Autodesk Inventor part; units mm, degrees
ref_plane "YZ Plane" through (0, 0, 0) normal (1, 0, 0) x (0, 1, 0)
ref_plane "XZ Plane" through (0, 0, 0) normal (0, 1, 0) x (-1, 0, 0)
ref_plane "XY Plane" through (0, 0, 0) normal (0, 0, 1) x (1, 0, 0)
sketch "Sketch1" plane through (0, 0, 0) normal (0, 0, 1) x (1, 0, 0)
  circle A0 centre (0, 0) radius 12.2936
  dimension "d0" = 24.5872
extrude "Extrusion1" add sketch "Sketch1" along normal blind 18.796
sketch "Sketch2" plane through (0, 0, 18.796) normal (0, 0, 1) x (1, 0, 0)
  circle A0 centre (0, 0) radius 12.2936
  circle A1 centre (0, 0) radius 3.4036
  circle A2 centre (0, 0) radius 1.905
  dimension "d3" = 6.8072
  dimension "d6" = 3.81
extrude "Extrusion3" add sketch "Sketch2" along normal blind 2.6162 contours A1
sketch "Sketch3" plane through (0, 0, 18.796) normal (0, 0, 1) x (1, 0, 0)
  circle A0 centre (0, 0) radius 12.2936
  point P0 (0, 8.5725)
  point P1 (0, -8.5725)
  dimension "d9" = 17.145
  dimension "d10" = 8.5725
hole "Hole1" at (0, 8.5725, 18.796) at (0, -8.5725, 18.796) direction (0, 0, -1) diameter 2.4638 depth 2.794 tip angle 118
sketch "Sketch4" plane through (0, 0, 0) normal (0, 0, -1) x (-1, 0, 0)
  circle A0 centre (0, 0) radius 12.2936
  circle A1 centre (0, 0) radius 11.8618
  dimension "d18" = 23.7236
extrude "Extrusion4" add sketch "Sketch4" along normal blind 30.5816 contours A1
sketch "Sketch5" plane through (0, 0, -30.5816) normal (0, 0, -1) x (-1, 0, 0)
  circle A0 centre (0, 0) radius 11.8618
  circle A1 centre (0, 0) radius 4.1148
  dimension "d21" = 8.2296
extrude "Extrusion5" add sketch "Sketch5" along normal blind 1.905 contours A1
sketch "Sketch6" plane through (0, 0, -32.4866) normal (0, 0, -1) x (-1, 0, 0)
  circle A0 centre (0, 0) radius 4.1148
  line L0 (-1.9805, -3.6068) -> (1.9805, -3.6068)
  dimension "d24" = 3.6068
  dimension "d25" = 8.2296
extrude "Extrusion6" cut sketch "Sketch6" against normal up to surface (1.905 mm away) contours L0 A0 picked at (-0.407, -3.7143)
sketch "Sketch7" plane through (0, 0, -32.4866) normal (0, 0, -1) x (-1, 0, 0)
  arc A0 (1.9805, -3.6068) -> (-1.9805, -3.6068) centre (0, 0) ccw
  circle A1 centre (0, 0) radius 0.9906
  dimension "d28" = 1.9812
extrude "Extrusion7" add sketch "Sketch7" along normal blind 0.889
sketch "Sketch8" plane through (0, 0, -30.5816) normal (0, 0, -1) x (-1, 0, 0)
  arc A0 (1.9805, -3.6068) -> (-1.9805, -3.6068) centre (0, 0) ccw
  line L0 (-8.6614, 1.5113) -> (-8.4328, 1.5113)
  line L1 (-8.4328, 1.5113) -> (-8.4328, -1.5113)
  line L2 (-8.4328, -1.5113) -> (-8.6614, -1.5113)
  line L3 (-8.6614, -1.5113) -> (-8.6614, 1.5113)
  line L4 (8.4328, 1.5113) -> (8.6614, 1.5113)
  line L5 (8.6614, 1.5113) -> (8.6614, -1.5113)
  line L6 (8.6614, -1.5113) -> (8.4328, -1.5113)
  line L7 (8.4328, -1.5113) -> (8.4328, 1.5113)
  point P0 (-8.4328, 0)
  point P1 (8.4328, 0)
  dimension "d31" = 0.2286
  dimension "d32" = 16.8656
  dimension "d33" = 3.0226
  dimension "d34" = 8.4328
extrude "Extrusion8" add sketch "Sketch8" along normal blind 6.096
sketch "Sketch9" plane through (8.6614, -1.5113, -30.5816) normal (1, 0, 0) x (0, 0, -1)
  line L0 (0, 0) -> (0, 3.0226)
  line L1 (0, 0) -> (6.096, 0)
  line L2 (6.096, 3.0226) -> (6.096, 0)
  line L3 (0, 3.0226) -> (6.096, 3.0226)
  arc A0 (4.7498, 0) -> (4.7498, 3.0226) centre (4.5746, 1.5113) ccw
  point P0 (-30.5816, 1.5113)
  dimension "d37" = 1.3462
extrude "Extrusion9" cut sketch "Sketch9" against normal through all contours A0 L2 L1 | L3 L2 A0
sketch "Sketch10" plane through (8.6614, -1.5113, -30.5816) normal (1, 0, 0) x (0, 0, -1)
  arc A0 (4.7498, 0) -> (4.7498, 3.0226) centre (4.5746, 1.5113) ccw
  line L0 (0, 0) -> (4.7498, 0)
  arc A1 (4.7747, 0.9652) -> (4.7747, 2.0574) centre (4.5746, 1.5113) ccw
  line L1 (3.6073, 0.9652) -> (4.7747, 0.9652)
  line L2 (3.6073, 2.0574) -> (4.7747, 2.0574)
  arc A2 (3.6073, 2.0574) -> (3.6073, 0.9652) centre (3.8074, 1.5113) ccw
  point P0 (-30.5816, 1.5113)
  dimension "d41" = 0.9398
  dimension "d42" = 0.5816
  dimension "d45" = 0.9652
  dimension "d46" = 0.5816
  dimension "d47" = 1.9304
extrude "Extrusion10" cut sketch "Sketch10" against normal through all
sketch "Sketch11" plane through (0, 0, 18.796) normal (0, 0, 1) x (1, 0, 0)
  circle A0 centre (0, 0) radius 12.2936
  circle A1 centre (-8.3693, 0) radius 2.3622
  circle A2 centre (8.3693, 0) radius 2.3622
  dimension "d50" = 4.7244
  dimension "d51" = 12.0142
  dimension "d53" = 16.7386
  dimension "d54" = 8.3693
extrude "Extrusion11" cut sketch "Sketch11" against normal blind 0.8636 contours A1 | A2
equation "\"d46\" = d42"
equation "\"d54\" = 0.5 * d53"
properties part number "Motor Body"
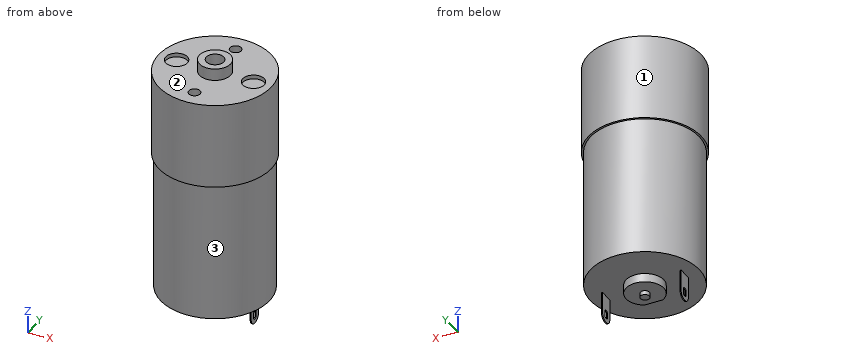
Here's how the part is built. I have some questions about the finished solid (model axes, mm). Face numbers are marked on the shaded views. A direction names the side the tool comes from. Round coordinates to 2 decimals unless told otherwise and drop trailing zeros. Order: outer loops, then holes, each group sorted by start corner. A loop starts at its lowest first (then second) coordinate and runs counter-clockwise, first axis right, second up. Notation, with made-up numbers: (68.5, -31) -> (125.5, -31) arc R28 cw to (125.5, 1) -> close; hole circle Ø11 at (79.5, 67). An arc over 180 degrees is marked (long way). Use a Markdown table: item, result. Add a question column.
(1) For the marked faces 1, 2 and 3, which set-ups out of +Z, -Z, +X, -X, +Y, -Y let a thin tool reach every point of the face, with its end or its side?
(2) I need wall thicknesses on line 1 along Z through (x, y) = (-2.5, 10); line 2 along Y through (x, z) = (0, -30.5); line 3 along Z through (x, y) = (-1.25, 3). Which ranges of each line are inside material? Lowest first, please.
(3) Suppose I cut it at C-C, the plane y = -4.5. Please give me the cut outline in (x, z).
(4) For pin 1 Ø2 at (x, y) = (-0.5, 6) entering from +Z; pin 2 Ø2.5 at (x, y) = (0, 0) entering from -Z; pin 3 Ø1 at (x, z) = (-4.5, 11.5) entering from +Y, each with a flat end and sliding along its axis, tell me the tip position at first contact or that it passes through.
(5) Suppose I cut it at D-D, the plane z = 4. Please give me the cut outline in (x, y).
(6) Suppose I cut it at A-A, the plane y = 0. Count the separate pieces of the cut face and the enclosed holes in it, and give its area (3 significant figures).
(7) Suppose I cut it at B-B, the plane x = -5. Please give me the cut outline in (y, z), and give its area (3 significant figures).
Verdict:
| question | item | result |
|---|---|---|
| 1 | face 1 | +Z, -Z |
| 1 | face 2 | +Z |
| 1 | face 3 | -Z |
| 2 | line 1 | -30.58 to 18.8 |
| 2 | line 2 | -11.86 to 11.86 |
| 2 | line 3 | -32.49 to 21.41 |
| 3 | outline | (-11.44, 0) -> (-10.98, 0) -> (-10.98, -30.58) -> (10.98, -30.58) -> (10.98, 0) -> (11.44, 0) -> (11.44, 18.8) -> (-11.44, 18.8) -> close |
| 4 | pin 1 | z = 18.8 |
| 4 | pin 2 | z = -33.38 |
| 4 | pin 3 | y = 11.62 |
| 5 | outline | circle Ø24.59 at (0, 0) |
| 6 | separate pieces | 3 |
| 6 | enclosed holes | 0 |
| 6 | area | 1,210 mm2 |
| 7 | outline | (-11.23, 0) -> (-10.76, 0) -> (-10.76, -30.58) -> (10.76, -30.58) -> (10.76, 0) -> (11.23, 0) -> (11.23, 18.8) -> (-11.23, 18.8) -> close |
| 7 | area | 1,080 mm2 |
